The listing builds one solid part. Answer for the finished solid, in the listing's coordinates (mm). A direction names the side the tool comes from. Round coordinates to 2 decimals unless told otherwise and drop trailing zeros. Write each loop counter-clockwise with the first axis right and the second up, starting at its lowest first coordinate (ties: lowest second). Pieces come first, ordered by that corner, then holes.
(1) A cutting plane is placed at C-C, the plane y = -19.5. Give the vertices of the cut face in (x, z), and give its area (3 significant figures).
(2) A cutting plane is placed at D-D, the plane z = 6. Give the vertices of the cut face in (x, y).
(3) For faces 4 (the face through (-4.32, -20.517, -17.372)), 5 (the face through (0, 5, 0)), determine the directions among +Z, -Z, +X, -X, +Y, -Y from which every point of the face is accessible in a straight line to the end or side of a thin tool.
(4) A cutting plane is placed at A-A, the plane z = -5. Give the vertices of the cut face in (x, y).
(5) Each of these flat-tipped pins is pushed along its axis until it touches: pin 1 Ø1 at (x, z) = (7, -4.5) entering from -Y; pin 2 Ø1 at (x, z) = (-3.5, -12) entering from -Y; pin 3 Ø3 at (x, y) = (6.5, -23) entering from +Z. Where does it stop, or does it pass through?
(6) The mould has two halves that part along Z. Classify faces 1 (the face through (0.161, -1.203, -13.555)), 2 (the face through (-5.7, 2.5, -6.6)), 3 (the face through (-9.5, -7, -16)): +Z half, -Z half, draft (parallel to the pull), parting line (faces both ways), or undercut.
(7) Find the intervals of material crossed by probe 1 along X at (y, z) = (3, 5); probe 2 along X at (y, z) = (3.95, -5); probe 3 along Y at (x, z) = (-2.75, -8.5), in increasing order.
(8) A cutting plane is placed at B-B, the plane x = -4.5. Give the number of separate pieces and of enclosed holes in the cut face, and give its area (3 significant figures).
from build123d import *

# Parameters (mm, degrees)
SKETCH1_W           = 19
SKETCH1_H           = 40
BOSS_EXTRUDE1_DEPTH = 5
CUT_EXTRUDE1_DEPTH  = 23.699118926
BOSS_EXTRUDE2_DEPTH = 35
SKETCH5_R           = 2
CUT_EXTRUDE2_DEPTH  = 46.719251962
SKETCH6_R           = 2
CUT_EXTRUDE3_DEPTH  = 54.870648729
FILLET1_R           = 4


with BuildPart() as part:
    # Sketch1 → Boss-Extrude1 (new body)
    with BuildSketch(Plane(origin=(0, 0, 0), x_dir=(1, 0, 0), z_dir=(0, 1, 0))):
        Rectangle(SKETCH1_W, SKETCH1_H)
    extrude(amount=BOSS_EXTRUDE1_DEPTH)

    # Sketch2 → Cut-Extrude1 (cut, through all)
    with BuildSketch(Plane(origin=(0, 5, 0), x_dir=(1, 0, 0), z_dir=(0, 1, 0))):
        Polygon((-9.5, 20), (9.5, 20), (9.5, 19.402900945), align=None)
    extrude(amount=-CUT_EXTRUDE1_DEPTH, mode=Mode.SUBTRACT)

    # Sketch4 → Boss-Extrude2 (add)
    with BuildSketch(Plane.XZ):
        Polygon((9.5, -19.402900945), (-9.5, -20), (-9.5, -15), (9.5, -14.402900945), align=None)
    extrude(amount=BOSS_EXTRUDE2_DEPTH)

    # Sketch5 → Cut-Extrude2 (cut, through all)
    with BuildSketch(Plane(origin=(0, 5, 0), x_dir=(1, 0, 0), z_dir=(0, 1, 0))):
        with Locations(Location((-4.5, 5, 0), (0, 0, 270))):
            Circle(SKETCH5_R)
        with Locations(Location((4.5, -5, 0), (0, 0, 270))):
            Circle(SKETCH5_R)
    extrude(amount=-CUT_EXTRUDE2_DEPTH, mode=Mode.SUBTRACT)

    # Sketch6 → Cut-Extrude3 (cut, through all)
    with BuildSketch(Plane(origin=(0.618532155, 0, -19.682012317), x_dir=(-0.9995065603657318, 0, -0.03141075907812129), z_dir=(0.03141075907812129, 0, -0.9995065603657318))):
        with Locations((-3.885852476, -12.5)):
            Circle(SKETCH6_R)
        with Locations((5.123527505, -22.5)):
            Circle(SKETCH6_R)
    extrude(amount=-CUT_EXTRUDE3_DEPTH, mode=Mode.SUBTRACT)

    # Fillet1
    fillet1_edges = [part.edges().sort_by_distance(p)[0] for p in [
        (0, 0, -14.701450473),
    ]]
    fillet(fillet1_edges, radius=FILLET1_R)


solid = part.part
Solutions:
1. outline: (-9.5, -20) - (9.5, -19.4) - (9.5, -14.4) - (-9.5, -15) - close
1. area: 95.0 mm2
2. outline: (-9.5, 0) - (2.77, 0) - (2.77, 5) - (-9.5, 5) - close; (6.23, 0) - (9.5, 0) - (9.5, 5) - (6.23, 5) - close
3. face 4: none
3. face 5: +Z, -Z, +X, -X, +Y
4. outline: (-9.5, 0) - (-6.5, 0) - (-6.5, 5) - (-9.5, 5) - close; (-2.5, 0) - (9.5, 0) - (9.5, 5) - (-2.5, 5) - close
5. pin 1: stops at y = 0
5. pin 2: stops at y = -0.37
5. pin 3: stops at z = -14.45
6. face 1: +Z half
6. face 2: undercut
6. face 3: draft
7. probe 1: x = -9.5 to 2.5, 6.5 to 9.5
7. probe 2: x = -9.5 to -6.5, -2.5 to 9.5
7. probe 3: y = 0 to 5
8. separate pieces: 3
8. enclosed holes: 0
8. area: 338 mm2
